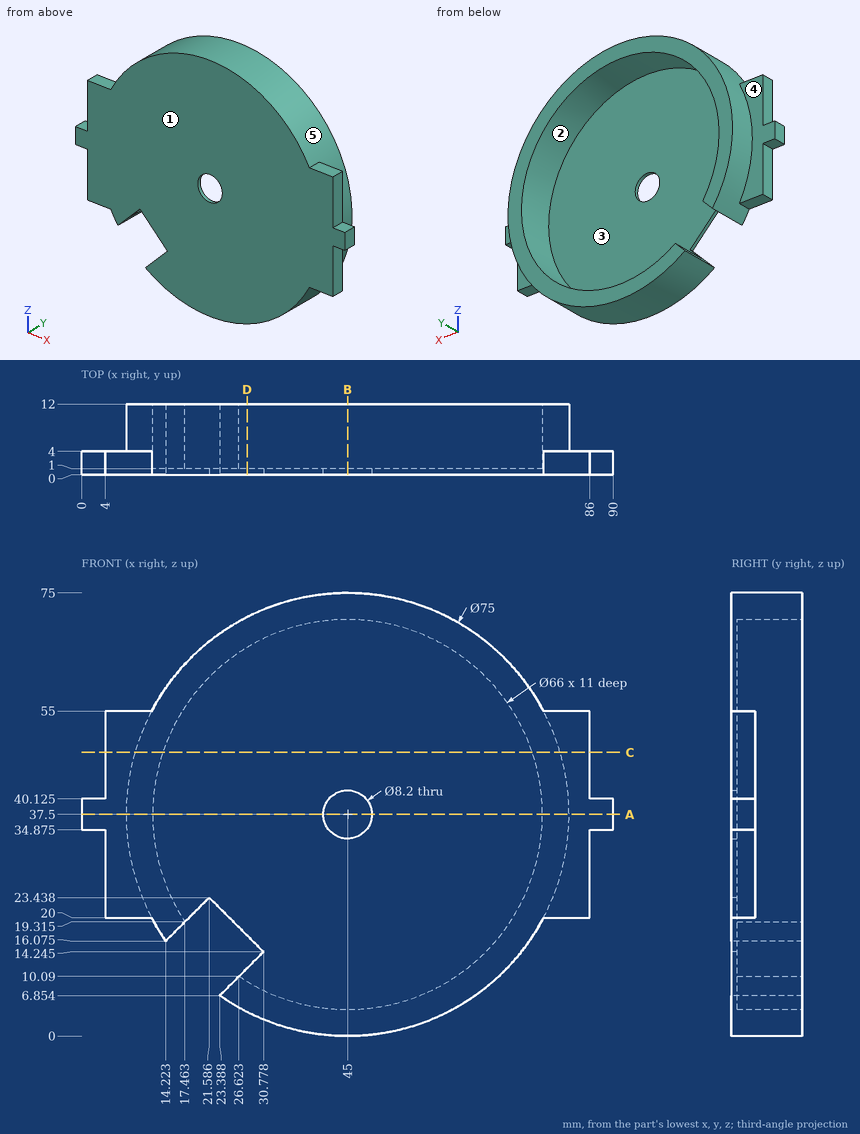
Can you work these out from the drawing? Everything is in mm from the part's minimum corner. A direction names the side the tool comes from. Round coordinates to 2 decimals unless told otherwise and drop trailing zeros. Order: outer loops, then holes, each group sorted by start corner. A loop starts at its lowest first (then second) coordinate and runs counter-clockwise, first axis right, second up. Notation, with made-up numbers: (30, 20) -> (64, 20) arc R23 ccw to (64, 46) -> close; hole circle Ø4 at (36.5, 81). An arc over 180 degrees is marked (long way). Return JSON: item names as keys, results as strings. Group by question number.
1. We'd pull the mould along X, two halves only. Please class the marked faces 3, 4 and 5: released by +X, released by -X, zero draft, split by the parting line, or undercut.
2. Will these pins go through, and if not, where does the flat tip stop? pin 1 (2 mm diameter, centred on x = 82, y = 1.5, fed in from +Z); pin 2 (1.5 mm diameter, centred on x = 65.5, z = 52.5, fed in from +Y); pin 3 (2 mm diameter, centred on x = 2.5, y = 1.5, fed in from -Z) (1 decimal).
3. If we section it at B-B, the plane x = 45: Write out the boundary of the cut face in (y, z), then the cut area to 3 significant figures.
4. If we section it at D-D, the plane x = 28: Write out the boundary of the cut face in (y, z) (1 decimal).
5. Which directions (+Z, -Z, +X, -X, +Y, -Y) give clear straight access to the entire face, cutting with the end or side of a thin tool? Please do the marked faces 1 and 2.
6. If we section it at A-A, the plane z = 37.5: Write out the boundary of the cut face in (x, y).
7. I need wall thicknesses on line 1 (Z direction, x = 45, y = 6.75); line 2 (Z direction, x = 45, y = 0.65); line 3 (X direction, y = 4.5, z = 37.5). Which ranges of each line are inside material? Lowest first, please. Write a range as [from, to].
8. If we section it at C-C, the plane z = 48: Write out the boundary of the cut face in (x, y) (1 decimal).
Output values:
{
 "1": {"face 3": "undercut", "face 4": "zero draft", "face 5": "split by the parting line"},
 "2": {"pin 1": "z = 55", "pin 2": "y = 1", "pin 3": "z = 34.9"},
 "3": {"outline": "(0, 0) -> (12, 0) -> (12, 4.5) -> (1, 4.5) -> (1, 33.4) -> (0, 33.4) -> close; (0, 41.6) -> (1, 41.6) -> (1, 70.5) -> (12, 70.5) -> (12, 75) -> (0, 75) -> close", "area": "166 mm²"},
 "4": {"outline": "(0, 4.1) -> (12, 4.1) -> (12, 9.2) -> (1, 9.2) -> (1, 11.5) -> (0, 11.5) -> close; (0, 17) -> (1, 17) -> (1, 65.8) -> (12, 65.8) -> (12, 70.9) -> (0, 70.9) -> close"},
 "5": {"face 1": "+Z, -Z, +X, -X, -Y", "face 2": "+Y"},
 "6": {"outline": "(0, 0) -> (40.9, 0) -> (40.9, 1) -> (12, 1) -> (12, 12) -> (7.5, 12) -> (7.5, 4) -> (0, 4) -> close; (49.1, 0) -> (90, 0) -> (90, 4) -> (82.5, 4) -> (82.5, 12) -> (78, 12) -> (78, 1) -> (49.1, 1) -> close"},
 "7": {"line 1": "[0, 4.5], [70.5, 75]", "line 2": "[0, 33.4], [41.6, 75]", "line 3": "[7.5, 12], [78, 82.5]"},
 "8": {"outline": "(4, 0) -> (86, 0) -> (86, 4) -> (81, 4) -> (81, 12) -> (76.3, 12) -> (76.3, 1) -> (13.7, 1) -> (13.7, 12) -> (9, 12) -> (9, 4) -> (4, 4) -> close"}
}
